Autodesk Fusion 360 part; units mm, degrees
sketch "Sketch1" plane through (0, 0, 0) normal (1, 0, 0) x (0, 1, 0)
  circle A0 centre (0, 0) radius 45
  line L0 (27.4205, -45) -> (-27.5795, -45)
  line L1 (-27.5795, -45) -> (-27.5795, -30)
  line L2 (-27.5795, -30) -> (27.4205, -30)
  line L3 (27.4205, -30) -> (27.4205, -45)
  dimension "d8" = 90
  dimension "d10" = 55
  dimension "d11" = 15
cylinder "CylinderPrimitive1" add diameter 90 height 13 placed x (0, 0, -1) y (0, 1, 0) z (1, 0, 0) at (0, 0, 0) makes body 1
fillet "Fillet1" radius 10 1 edges at (13, -16.2727, 41.9547) on bodies 1
extrude "Extrude1" add sketch "Sketch1" along normal blind 13 contours A0 L1 L2 L3 | A0 L0 L1 | A0 L0 L3 picked at (-0.053, -35) bodies 1
cylinder "CylinderPrimitive2" add diameter 90 height 13 placed x (0, 0, 1) y (0, 1, 0) z (-1, 0, 0) at (0, 0, 0) bodies 1
fillet "Fillet2" radius 10 1 edges at (-13, -16.2727, -41.9547) on bodies 1
extrude "Extrude2" add sketch "Sketch1" against normal blind 13 contours A0 L1 L2 L3 | A0 L0 L1 | A0 L0 L3 picked at (-0.053, -35) bodies 1
ref_plane "WorkPlane1" through (-0.4102, 0, 45) normal (0, 0, 1) x (0, 1, 0)
sketch "Sketch5" plane through (-0.4102, 0, 45) normal (0, 0, 1) x (1, 0, 0)
  circle A0 centre (0, 0) radius 12
  dimension "d26" = 24
extrude "Extrude3" add sketch "Sketch5" against normal blind 10 bodies 1
extrude "Extrude4" add 1 faces at (0.1622, 3.9888, 45) along direction (0, 0, 1) blind 22 on bodies 1 bodies 1
copy_body "Body->Comp1" bodies 1 removing the originals makes body 2 in component "Component"
component "Component" placed x (1, 0, 0) y (0, 1, 0) z (0, 0, 1) at (0, 0, 0)
equation "start_dia = 80 mm"
equation "diameter = 90 mm"
equation "base_length = 55 mm"
equation "base_depth = 26 mm"
equation "top_dia = 24 mm"
equation "top_length = 22 mm"
equation "base_height = 15 mm"
equation "d8 = diameter"
equation "d10 = base_length"
equation "d11 = base_height"
equation "d12 = base_depth / 2"
equation "d16 = diameter - start_dia"
equation "d17 = base_depth / 2"
equation "d19 = base_depth / 2"
equation "d23 = -base_depth / 2"
equation "d26 = top_dia"
equation "d29 = top_length"
Can you work these out from the model? Positions are in its coordinate system, mm. A direction names the side the tool comes from. Round coordinates to 2 decimals unless told otherwise and drop trailing zeros. Loops run counter-clockwise (first coordinate to the right, second up) from the corner with the lowest first, then second, coordinate; pieces in that order, holes last. Notation, with made-up numbers: (-1.5, 52) -> (51.5, 52) arc R34 ccw to (51.5, 85) -> close; hole circle Ø1 at (-26, -18.75). An arc over 180 degrees is marked (long way). Answer in a Markdown table with one row per item.
Item 1: On a 3-axis mill with a long thin cutter (end or side, diameter ignored), from which of +Z, -Z, +X, -X, +Y, -Y can I reach the whole of each face in a straight line? I mean faces 1 (the flat face through (-13, 0, -6)), 2 (the cylindrical face through (-12.4, -0.5, 55.7)). Say none if no direction works.
Answer block:
| item | result |
|---|---|
| face 1 | +Z, -Z, -X, +Y, -Y |
| face 2 | +Z |
Item 2: If I drill on probe 1 along Y at (x, z) = (9.5, 22); probe 2 along Z at (x, y) = (-9.75, -10.5); probe 3 along Z at (x, y) = (10.25, -29.5), over which ranges is the centre line in solid material (lowest first)?
Answer block:
| item | result |
|---|---|
| probe 1 | -36.48 to 36.48 |
| probe 2 | -45 to 41.06 |
| probe 3 | -29.74 to 29.74 |
Item 3: Suppose I cut it at C-C, the plane y = 0. List the corners of the cut face in (x, z) for me, plus the area to 3 significant figures.
Answer block:
| item | result |
|---|---|
| outline | (-13, -45) -> (13, -45) -> (13, 35) arc R10 ccw to (11.59, 40.12) -> (11.59, 67) -> (-12.41, 67) -> (-12.41, 38.38) arc R10 ccw to (-13, 35) -> close |
| area | 2,850 mm² |
Item 4: Suppose I cut it at A-A, the plane x = -6. List the corners of the cut face in (y, z) for me, plus the area to 3 significant figures.
Answer block:
| item | result |
|---|---|
| outline | (-27.58, -45) -> (27.42, -45) -> (27.42, -35.1) arc R44.54 ccw to (10.62, 43.26) -> (10.62, 67) -> (-10.62, 67) -> (-10.62, 43.26) arc R44.54 ccw to (-27.58, -34.97) -> close |
| area | 6,910 mm² |
Item 5: Suppose I cut it at B-B, the plane z = 56. List the corners of the cut face in (x, y) for me.
Answer block:
| item | result |
|---|---|
| outline | circle Ø24 at (-0.41, 0) |
Item 6: Will these pins go through, and if not, where does the flat tip stop? P1, Ø2, axis at x = 11.5, y = -21.5, coming from the +Z side; P2, Ø2, axis at x = 3, z = 37.5, coming from the -Y side; P3, Ø3, axis at x = 7.5, z = 16.5, coming from the +Y side; P4, Ø6, axis at x = 4.5, y = 13.5, coming from the +Z side.
Answer block:
| item | result |
|---|---|
| P1 | z = 35.76 |
| P2 | y = -26.32 |
| P3 | y = 41.62 |
| P4 | z = 67 |
